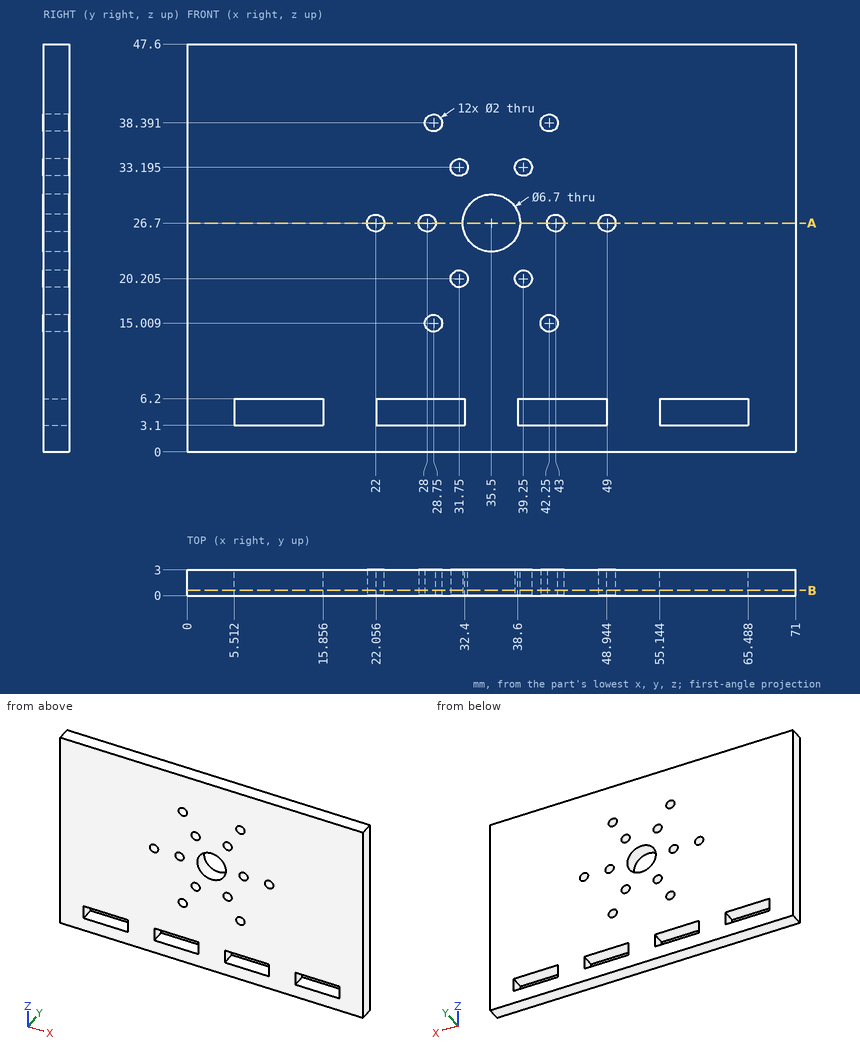
Verification items for this drawing (mm, ordinates from the low corner). Coordinates: 2 decimals unless noted, no trailing zeros. Loops run counter-clockwise (first coordinate to the right, second up) from the corner with the lowest first, then second, coordinate; pieces in that order, holes last. Notation, with made-up numbers: (89.5, 64.25) -> (94.5, 64.25) arc R22 ccw to (94.5, 78.25) -> close; hole circle Ø9 at (0.25, 80). An arc over 180 degrees is marked (long way). Answer in a Markdown table with one row per item. Add a question column.
1. Material ranges on probe 1 along X at (y, z) = (2.8, 5.5); probe 2 along Z at (x, y) = (39.25, 2.4) (1 decimal); probe 3 along Z at (x, y) = (42.25, 0.8), recorded low to high. Write a range as [from, to].
2. Section check B-B, the plane y = 0.6. Give the number of separate pieces and of enclosed holes in the cut face, then the cut area to 3 significant figures.
3. Section check A-A, the plane z = 26.7. Enter the section's corners in (x, y), then the cut area to 3 significant figures.
Derived:
| question | item | result |
|---|---|---|
| 1 | probe 1 | x = [0, 5.51], [15.86, 22.06], [32.4, 38.6], [48.94, 55.14], [65.49, 71] |
| 1 | probe 2 | z = [0, 3.1], [6.2, 19.2], [21.2, 32.2], [34.2, 47.6] |
| 1 | probe 3 | z = [0, 3.1], [6.2, 14.01], [16.01, 26.04], [27.36, 37.39], [39.39, 47.6] |
| 2 | separate pieces | 1 |
| 2 | enclosed holes | 17 |
| 2 | area | 3,180 mm² |
| 3 | outline | (0, 0) -> (21, 0) -> (21, 3) -> (0, 3) -> close; (23, 0) -> (27, 0) -> (27, 3) -> (23, 3) -> close; (29, 0) -> (32.15, 0) -> (32.15, 3) -> (29, 3) -> close; (38.85, 0) -> (42, 0) -> (42, 3) -> (38.85, 3) -> close; (44, 0) -> (48, 0) -> (48, 3) -> (44, 3) -> close; (50, 0) -> (71, 0) -> (71, 3) -> (50, 3) -> close |
| 3 | area | 169 mm² |
